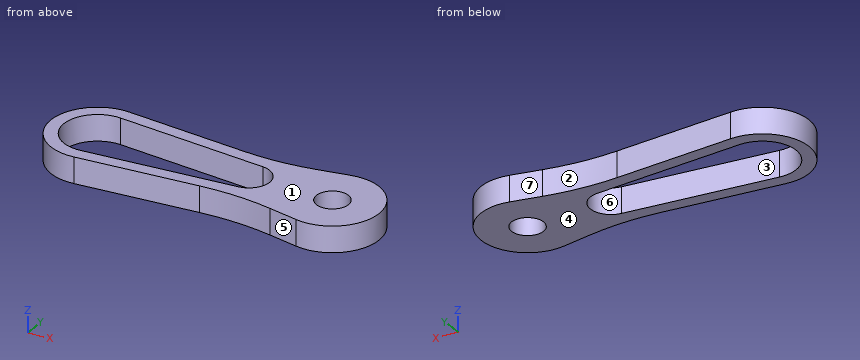
from build123d import *

# Parameters (mm, degrees)
TIJELO_DEPTH       = 5
UTOR_ZA_RUKU_DEPTH = 55.972720508
SKETCH8_R          = 3.1
CUT_EXTRUDE2_DEPTH = 10


with BuildPart() as part:
    # Sketch2 → Tijelo (new body)
    with BuildSketch(Plane.XY):
        with BuildLine():
            Line((0.775862069, 8.966495305), (23.705382946, 6.98242629))
            ThreePointArc((23.705382946, 6.98242629), (30.68412811, 6.867543469), (37.610875669, 7.725593798))
            Line((37.610875669, 7.725593798), (43.272873379, 8.832725153))
            ThreePointArc((43.272873379, 8.832725153), (54, 0), (43.272873379, -8.832725153))
            Line((43.272873379, -8.832725153), (37.610875669, -7.725593798))
            ThreePointArc((37.610875669, -7.725593798), (30.68412811, -6.867543469), (23.705382946, -6.98242629))
            Line((23.705382946, -6.98242629), (0.775862069, -8.966495305))
            ThreePointArc((0.775862069, -8.966495305), (-9, 0), (0.775862069, 8.966495305))
        make_face()
    extrude(amount=TIJELO_DEPTH)

    # Sketch1 → Utor za ruku (cut, through all)
    with BuildSketch(Plane.XY):
        with BuildLine():
            Line((0.560344828, 6.475802165), (29.344827586, 3.985109024))
            ThreePointArc((29.344827586, 3.985109024), (33, 0), (29.344827586, -3.985109024))
            Line((29.344827586, -3.985109024), (0.560344828, -6.475802165))
            ThreePointArc((0.560344828, -6.475802165), (-6.5, 0), (0.560344828, 6.475802165))
        make_face()
    extrude(amount=UTOR_ZA_RUKU_DEPTH, mode=Mode.SUBTRACT)

    # Sketch8 → Cut-Extrude2 (cut)
    with BuildSketch(Plane.XY):
        with Locations((45, 0)):
            Circle(SKETCH8_R)
    extrude(amount=CUT_EXTRUDE2_DEPTH, mode=Mode.SUBTRACT)


solid = part.part
Geometry check sheet. Reference: the model listing, model coordinates, mm. Face numbers are marked on the shaded views. A direction names the side the tool comes from. Give positions to 0.01 mm unless a question says otherwise; leave off trailing zeros. Order: outer loops, then holes, each group sorted by start corner. A loop starts at its lowest first (then second) coordinate and runs counter-clockwise, first axis right, second up.
1) Gauge pin test, flat ends, axial feed: pin 1 (2 mm diameter, centred on y = -2.5, z = 3.5, fed in from -X); pin 2 (3 mm diameter, centred on x = 34, z = 4.5, fed in from -Y). Record the tip position at first contact, or that the pin passes through.
Results are:
pin 1: stops at x = -8.87
pin 2: stops at y = -7.36
2) Draft check along Y on the marked faces 1, 2 and 3. Enter one of: released by +Y, released by -Y, zero draft, split by the parting line, or undercut.
Results are:
face 1: zero draft
face 2: released by +Y
face 3: undercut
3) Cross-section at B-B (x = 0). Record the boundary of the cut face in (y, z).
Results are:
outline: (-9, 0) - (-6.5, 0) - (-6.5, 5) - (-9, 5) - close; (6.5, 0) - (9, 0) - (9, 5) - (6.5, 5) - close
4) Cross-section at A-A (y = 0). Record the boundary of the cut face in (x, z).
Results are:
outline: (-9, 0) - (-6.5, 0) - (-6.5, 5) - (-9, 5) - close; (33, 0) - (41.9, 0) - (41.9, 5) - (33, 5) - close; (48.1, 0) - (54, 0) - (54, 5) - (48.1, 5) - close
5) Cross-section at C-C (z = 2.05). Record the boundary of the cut face in (x, y), then the cut area to 3 significant figures.
Results are:
outline: (0.78, -8.97) - (23.71, -6.98) arc R50 cw to (37.61, -7.73) - (43.27, -8.83) arc R9 ccw (long way) to (43.27, 8.83) - (37.61, 7.73) arc R50 cw to (23.71, 6.98) - (0.78, 8.97) arc R9 ccw (long way) to start; hole (0.56, -6.48) - (29.34, -3.99) arc R4 ccw to (29.34, 3.99) - (0.56, 6.48) arc R6.5 ccw (long way) to start; hole circle Ø6.2 at (45, 0)
area: 527 mm2
6) Cross-section at D-D (x = 45). Record the boundary of the cut face in (y, z).
Results are:
outline: (-9, 0) - (-3.1, 0) - (-3.1, 5) - (-9, 5) - close; (3.1, 0) - (9, 0) - (9, 5) - (3.1, 5) - close
7) Tool access check on the marked faces 4, 5, 6 and 7. Record the directions out of +Z, -Z, +X, -X, +Y, -Y that give a thin tool (end or side, any length) a straight path to the whole face; none if there is none.
Results are:
face 4: -Z, +X, -X, +Y, -Y
face 5: +Z, -Z, -Y
face 6: +Z, -Z
face 7: +Z, -Z, +Y
8) Material ranges on probe 1 along X at (y, z) = (0, 2.25); probe 2 along X at (y, z) = (-2.5, 4.4); probe 3 along Y at (x, z) = (0, 1.9), recorded low to high.
Results are:
probe 1: x = -9 to -6.5, 33 to 41.9, 48.1 to 54
probe 2: x = -8.65 to -6, 32.12 to 43.17, 46.83 to 53.65
probe 3: y = -9 to -6.5, 6.5 to 9
